from build123d import *

# Parameters (mm, degrees)
SKETCH1_R               = 23.5
BOSS_EXTRUDE1_DEPTH     = 112.5
SKETCH2_OUTSIDE_W       = 484.702
SKETCH2_OUTSIDE_H       = 522.81
SKETCH2_OUTSIDE_R       = 140
CUT_EXTRUDE2_DEPTH      = 80.5
SKETCH3_R               = 100
BOSS_EXTRUDE2_DEPTH     = 160
SKETCH5_R               = 37.5
BOSS_EXTRUDE3_DEPTH     = 325
SKETCH6_R               = 28.1
CUT_EXTRUDE3_DEPTH      = 310
SKETCH7_R               = 50
CUT_EXTRUDE4_DEPTH      = 25
SKETCH8_R               = 10.15
CUT_EXTRUDE5_DEPTH      = 15
CUT_EXTRUDE6_DEPTH      = 323.343674653
CUT_EXTRUDE6_DEPTH_BACK = 323.343674653
SKETCH9_R               = 97


with BuildPart() as part:
    # Sketch1 → Boss-Extrude1 (new, symmetric)
    with BuildSketch(Plane(origin=(0, 0, 0), x_dir=(1, 0, 0), z_dir=(0, 1, 0))):
        with BuildLine():
            Line((175, 50), (130.766968306, 50))
            ThreePointArc((130.766968306, 50), (70, 121.24355653), (-22.082213964, 138.247516529))
            Line((-22.082213964, 138.247516529), (-44.198729811, 176.554445662))
            ThreePointArc((-44.198729811, 176.554445662), (-112.5, 194.855715852), (-130.801270189, 126.554445662))
            Line((-130.801270189, 126.554445662), (-108.684754342, 88.247516529))
            ThreePointArc((-108.684754342, 88.247516529), (-140, 0), (-108.684754342, -88.247516529))
            Line((-108.684754342, -88.247516529), (-130.801270189, -126.554445662))
            ThreePointArc((-130.801270189, -126.554445662), (-112.5, -194.855715851), (-44.198729811, -176.554445662))
            Line((-44.198729811, -176.554445662), (-22.082213964, -138.247516529))
            ThreePointArc((-22.082213964, -138.247516529), (70, -121.24355653), (130.766968306, -50))
            Line((130.766968306, -50), (175, -50))
            ThreePointArc((175, -50), (225, 0), (175, 50))
        make_face()
        with Locations(Location((175, 0, 0), (0, 0, 270))):
            Circle(SKETCH1_R, mode=Mode.SUBTRACT)
        with Locations(Location((-87.5, 151.554445662, 0), (0, 0, 270))):
            Circle(SKETCH1_R, mode=Mode.SUBTRACT)
        with Locations(Location((-87.5, -151.554445662, 0), (0, 0, 270))):
            Circle(SKETCH1_R, mode=Mode.SUBTRACT)
    extrude(amount=BOSS_EXTRUDE1_DEPTH, both=True)

    # Sketch2 outside → Cut-Extrude2 (cut, symmetric)
    with BuildSketch(Plane(origin=(0, 0, 0), x_dir=(1, 0, 0), z_dir=(0, 1, 0))):
        with Locations((42.5, 0)):
            Rectangle(SKETCH2_OUTSIDE_W, SKETCH2_OUTSIDE_H)
        with Locations(Location((0, 0, 0), (0, 0, 99.075167572))):
            Circle(SKETCH2_OUTSIDE_R, mode=Mode.SUBTRACT)
    extrude(amount=CUT_EXTRUDE2_DEPTH, both=True, mode=Mode.SUBTRACT)

    # Sketch3 → Boss-Extrude2 (add)
    with BuildSketch(Plane(origin=(0, 0, 0), x_dir=(0, 0, -1), z_dir=(1, 0, 0))):
        Circle(SKETCH3_R)
    extrude(amount=-BOSS_EXTRUDE2_DEPTH)

    # Sketch5 → Boss-Extrude3 (add)
    with BuildSketch(Plane.ZY.offset(160)):
        Circle(SKETCH5_R)
    extrude(amount=-BOSS_EXTRUDE3_DEPTH)

    # Sketch6 → Cut-Extrude3 (cut)
    with BuildSketch(Plane.ZY.offset(160)):
        Circle(SKETCH6_R)
    extrude(amount=-CUT_EXTRUDE3_DEPTH, mode=Mode.SUBTRACT)

    # Sketch7 → Cut-Extrude4 (cut)
    with BuildSketch(Plane.ZY.offset(160)):
        Circle(SKETCH7_R)
    extrude(amount=-CUT_EXTRUDE4_DEPTH, mode=Mode.SUBTRACT)

    # Sketch8 → Cut-Extrude5 (cut)
    with BuildSketch(Plane.ZY.offset(160)):
        with Locations((0, 74.921014489)):
            Circle(SKETCH8_R)
        with Locations((64.951905284, -37.578985511)):
            Circle(SKETCH8_R)
        with Locations((-64.951905284, -37.578985511)):
            Circle(SKETCH8_R)
    extrude(amount=-CUT_EXTRUDE5_DEPTH, mode=Mode.SUBTRACT)

    # Sketch9 → Cut-Extrude6 (cut, two sides: drawn at the far end of the back side and taken through both)
    with BuildSketch(Plane(origin=(0, 0, 0), x_dir=(1, 0, 0), z_dir=(0, 1, 0)).offset(-CUT_EXTRUDE6_DEPTH_BACK)):
        with Locations(Location((0, 0, 0), (0, 0, 270))):
            Circle(SKETCH9_R)
    extrude(amount=CUT_EXTRUDE6_DEPTH + CUT_EXTRUDE6_DEPTH_BACK, mode=Mode.SUBTRACT)


solid = part.part
Source: CAD feature listing. Evaluate the final solid. Frame: model axes, mm. A direction names the side the tool comes from. Round coordinates to 2 decimals unless told otherwise and drop trailing zeros. Loops run counter-clockwise (first coordinate to the right, second up) from the corner with the lowest first, then second, coordinate; pieces in that order, holes last. Notation, with made-up numbers: M 87,45.5 L 111,45.5 A13 ccw 111,53.5 Z; hole C 12.25,37 d8. An arc over 180 degrees is marked long. Return JSON: item names as keys, results as strings. Group by question number.
1. Pin query (flat end, axial travel): pin 1 (6 mm diameter, centred on y = -40, z = -61.5, fed in from -X); pin 2 (9.5 mm diameter, centred on x = 152, y = 98.5, fed in from +Z); pin 3 (6 mm diameter, centred on y = -15.5, z = -41.5, fed in from -X); pin 4 (8 mm diameter, centred on x = 26.5, z = 144, fed in from -Y). Return the tip coordinate at first contact, or that it passes through.
2. Reachability of faces 5 (the face through (-119.588, -96.276, 107.133)), 6 (the face through (153, 97, 50)), 7 (the face through (-145, -37, 65)) from +Z, -Z, +X, -X, +Y, -Y: full face, straight path, thin tool, end or side. Return the list, or none.
3. Section query B-B on z = -156. Output: boundary loops of the cut face in (x, y), and give its area (3 significant figures).
4. Section query A-A on x = 0. Output: boundary loops of the cut face in (y, z), and give its area (4 significant figures).
5. Section query C-C on y = 0. Output: boundary loops of the cut face in (x, z).
6. Section query D-D on y = 93.5. Output: boundary loops of the cut face in (x, z), and give its area (3 significant figures).
7. Mould query, pull axis X, two halves, no side actions, for faces 1 (the face through (-96.501, -96.724, -129.846)), 2 (the face through (-145, -37, -65)), 3 (the face through (224.988, -96.276, 1.099)), 4 (the face through (-106, 80.5, -171)). Classes: released by +X, released by -X, zero draft, split by the parting line, or undercut.
8. Material intervals for line 1 along Y through (x, z) = (-156.25, 0); line 2 along X through (y, z) = (-101, 0); line 3 along Y through (x, z) = (-64, -163.5), sorted ascending. Write a range as from..to.
Checks:
{
 "1": {"pin 1": "stops at x = -145", "pin 2": "stops at z = 50", "pin 3": "stops at x = -135", "pin 4": "passes through"},
 "2": {"face 5": "-X, -Y", "face 6": "+Z, +X, +Y, -Y", "face 7": "-X"},
 "3": {"outline": "M -137.3,-112.5 L -110.58,-112.5 L -110.58,-80.5 L -137.3,-80.5 Z; M -137.3,80.5 L -110.58,80.5 L -110.58,112.5 L -137.3,112.5 Z; M -64.42,-112.5 L -32.33,-112.5 L -32.33,-80.5 L -64.42,-80.5 Z; M -64.42,80.5 L -32.33,80.5 L -32.33,112.5 L -64.42,112.5 Z", "area": "3,760 mm²"},
 "4": {"outline": "M -112.5,-140 L 112.5,-140 L 112.5,-97 L -112.5,-97 Z; M -112.5,97 L 112.5,97 L 112.5,140 L -112.5,140 Z", "area": "19,350 mm²"},
 "5": {"outline": "M -160,-100 L -97.98,-100 A140 ccw 134.88,-37.5 L 165,-37.5 L 165,37.5 L 134.88,37.5 A140 ccw -97.98,100 L -160,100 L -160,50 L -135,50 L -135,28.1 L -92.84,28.1 A97 cw 92.84,28.1 L 150,28.1 L 150,-28.1 L 92.84,-28.1 A97 cw -92.84,-28.1 L -135,-28.1 L -135,-50 L -160,-50 Z"},
 "6": {"outline": "M -160,-35.46 L -135.43,-35.46 A140 ccw -108.68,-88.25 L -130.8,-126.55 A50 ccw -44.2,-176.55 L -22.08,-138.25 A140 ccw 130.77,-50 L 175,-50 A50 ccw 175,50 L 130.77,50 A140 ccw -22.08,138.25 L -44.2,176.55 A50 ccw -130.8,126.55 L -108.68,88.25 A140 ccw -135.43,35.46 L -160,35.46 Z; hole C -87.5,-151.55 d47; hole C -87.5,151.55 d47; hole C 0,0 d194; hole C 175,0 d47", "area": "51,500 mm²"},
 "7": {"face 1": "undercut", "face 2": "released by -X", "face 3": "released by +X", "face 4": "zero draft"},
 "8": {"line 1": "y = -100..-50, 50..64.77, 85.07..100", "line 2": "x = -140..-97, 97..151.5, 198.5..225", "line 3": "y = -112.5..-80.5, 80.5..112.5"}
}
